from build123d import *

# Parameters (mm, degrees)
CROQUIS1_R              = 5.95
SALIENTE_EXTRUIR1_DEPTH = 5
CROQUIS2_R              = 5.375
SALIENTE_EXTRUIR2_DEPTH = 1
CROQUIS4_W              = 1.4
CROQUIS4_H              = 4.624223677
CROQUIS4_H_2            = 1.41
CROQUIS4_W_2            = 4.628564535
SALIENTE_EXTRUIR3_DEPTH = 70
REDONDEO1_R             = 1
CROQUIS5_R              = 5.375
SALIENTE_EXTRUIR4_DEPTH = 1.45


with BuildPart() as part:
    # Croquis1 → Saliente-Extruir1 (new body)
    with BuildSketch(Plane.XY):
        Circle(CROQUIS1_R)
    extrude(amount=SALIENTE_EXTRUIR1_DEPTH)

    # Croquis2 → Saliente-Extruir2 (add)
    with BuildSketch(Plane(origin=(0, 0, 0), x_dir=(-1, 0, 0), z_dir=(0, 0, -1))):
        Circle(CROQUIS2_R)
    extrude(amount=SALIENTE_EXTRUIR2_DEPTH)

    # Croquis4 → Saliente-Extruir3 (add)
    with BuildSketch(Plane(origin=(0, 0, -1), x_dir=(-1, 0, 0), z_dir=(0, 0, -1))):
        with Locations((0, 3.017111839)):
            Rectangle(CROQUIS4_W, CROQUIS4_H)
        Rectangle(CROQUIS4_W, CROQUIS4_H_2)
        with Locations((0, -3.017111839)):
            Rectangle(CROQUIS4_W, CROQUIS4_H)
        with Locations((-3.014282268, 0)):
            Rectangle(CROQUIS4_W_2, CROQUIS4_H_2)
        with Locations((3.014282268, 0)):
            Rectangle(CROQUIS4_W_2, CROQUIS4_H_2)
    extrude(amount=SALIENTE_EXTRUIR3_DEPTH)

    # Redondeo1
    redondeo1_edges = [part.edges().sort_by_distance(p)[0] for p in [
        (-5.95, 0, 5),
    ]]
    fillet(redondeo1_edges, radius=REDONDEO1_R)

    # Croquis5 → Saliente-Extruir4 (add)
    with BuildSketch(Plane(origin=(0, 0, -71), x_dir=(-1, 0, 0), z_dir=(0, 0, -1))):
        with Locations(Location((0, 0, 0), (0, 0, 172.4632093))):
            Circle(CROQUIS5_R)
    extrude(amount=SALIENTE_EXTRUIR4_DEPTH)


solid = part.part
Verification items for the finished model (mm, model axes). A direction names the side the tool comes from. Coordinates: 2 decimals unless noted, no trailing zeros. Order: outer loops, then holes, each group sorted by start corner. A loop starts at its lowest first (then second) coordinate and runs counter-clockwise, first axis right, second up. Notation, with made-up numbers: M 67.5,72 L 121.5,72 A13 ccw 121.5,87 Z; hole C 47,38.5 d10. An arc over 180 degrees is marked long. One line per item, written item: value. Start each with the question number.
Item 1: Access from +Z, -Z, +X, -X, +Y, -Y to the whole of each face (thin tool, end or side, straight path). Record for faces 3 (the flat face through (3, 2, -71)), 4 (the cylindrical face through (3.459, -4.114, -71.715)), 5 (the flat face through (-2, 3, -71)).
Item 2: Mould release check, pull along Z, two halves, no side actions. Record for faces 1 (the flat face through (-0.7, -3, -36)), 2 (the flat face through (0, 0, 5)): released by +Z, released by -Z, zero draft, split by the parting line, or undercut.
Item 3: Gauge pin test, flat ends, axial feed: pin 1 (2.5 mm diameter, centred on y = -3, z = -38.5, fed in from +X); pin 2 (4 mm diameter, centred on x = 3.5, z = -28, fed in from +Y) (3 decimals); pin 3 (1.6 mm diameter, centred on y = 0, z = -35.5, fed in from -X). Record the tip position at first contact, or that the pin passes through.
Item 4: Sectioned sample at A-A (z = -31). Enter the section's corners in (x, y) (3 decimals).
Item 5: Sectioned sample at B-B (x = 0). Enter the section's corners in (y, z) (3 decimals), then the cut area to 4 significant figures.
Item 6: Scan lines: probe 1 along Z at (x, y) = (3, -3.5); probe 2 along X at (y, z) = (3.5, -68); probe 3 along Y at (x, z) = (1.5, -34.5) (3 decimals). Record each from-to range of solid material in increasing order.
Conclusion:
1. face 3: +X, +Y
1. face 4: -Z
1. face 5: -X, +Y
2. face 1: undercut
2. face 2: released by +Z
3. pin 1: stops at x = 0.7
3. pin 2: stops at y = 0.705
3. pin 3: stops at x = -5.33
4. outline: M -5.329,-0.705 L -0.7,-0.705 L -0.7,-5.329 L 0.7,-5.329 L 0.7,-0.705 L 5.329,-0.705 L 5.329,0.705 L 0.7,0.705 L 0.7,5.329 L -0.7,5.329 L -0.7,0.705 L -5.329,0.705 Z
5. outline: M -5.95,0 L -5.375,0 L -5.375,-1 L -5.329,-1 L -5.329,-71 L -5.375,-71 L -5.375,-72.45 L 5.375,-72.45 L 5.375,-71 L 5.329,-71 L 5.329,-1 L 5.375,-1 L 5.375,0 L 5.95,0 L 5.95,4 A1 ccw 4.95,5 L -4.95,5 A1 ccw -5.95,4 Z
5. area: 831.5 mm^2
6. probe 1: z = -72.45 to -71, -1 to 5
6. probe 2: x = -0.7 to 0.7
6. probe 3: y = -0.705 to 0.705
